```python
from build123d import *

# Parameters (mm, degrees)
SKETCH1_W           = 50.8
SKETCH1_H           = 25.4
SKETCH1_W_2         = 47.752
SKETCH1_H_2         = 22.352
EXTRUDE_THIN1_DEPTH = 304.8
SKETCH2_R           = 14.2875
CUT_EXTRUDE2_DEPTH  = 25.4


with BuildPart() as part:
    # Sketch1 → Extrude-Thin1 (new body)
    with BuildSketch(Plane.XY):
        with Locations((-25.4, -12.7)):
            Rectangle(SKETCH1_W, SKETCH1_H)
        with Locations((-25.4, -12.7)):
            Rectangle(SKETCH1_W_2, SKETCH1_H_2, mode=Mode.SUBTRACT)
    extrude(amount=EXTRUDE_THIN1_DEPTH)

    # Sketch2 → Cut-Extrude2 (cut)
    with BuildSketch(Plane(origin=(0, 0, 0), x_dir=(1, 0, 0), z_dir=(0, 1, 0))):
        with Locations(Location((-25.4, -25.4, 0), (0, 0, 270))):
            Circle(SKETCH2_R)
    extrude(amount=-CUT_EXTRUDE2_DEPTH, mode=Mode.SUBTRACT)


solid = part.part
```
Verification items for the finished model (mm, model axes). A direction names the side the tool comes from. Coordinates: 2 decimals unless noted, no trailing zeros. Write each loop counter-clockwise with the first axis right and the second up, starting at its lowest first coordinate (ties: lowest second). Pieces come first, ordered by that corner, then holes. Notation, with made-up numbers: (21.25, 73) - (40.25, 73) arc R22 cw to (40.25, 108) - close; hole circle Ø4 at (3, 54.5). An arc over 180 degrees is marked (long way). One line per question, with ' | ' between items. Start each with the question number.
1. Section check C-C (x = -17). Enter the section's corners in (y, z).
2. Section check B-B (z = 25.4). Enter the section's corners in (x, y).
3. Draft check along Z on faces 3 (the flat face through (-26, -25, 0)), 4 (the cylindrical face through (-15.744, -0.751, 14.87)), 5 (the flat face through (0, -13, 150)). Enter one of: released by +Z, released by -Z, zero draft, split by the parting line, or undercut.
4. Section check D-D (z = 219). Enter the section's corners in (x, y).
5. Access from +Z, -Z, +X, -X, +Y, -Y to the whole of each face (thin tool, end or side, straight path). Record for faces 1 (the cylindrical face through (-15.744, -24.627, 14.87)), 2 (the flat face through (-26, -23.876, 150)).
6. Section check A-A (y = -20). Enter the section's corners in (x, z), plus the area to 3 significant figures.
7. Material ranges on line 1 along X through (y, z) = (-7.25, 81.5); line 2 along Y through (x, z) = (-11.5, 33); line 3 along X through (y, z) = (-24.95, 25.4), recorded low to high.
Computed values:
1) outline: (-25.4, 0) - (-23.88, 0) - (-23.88, 13.84) - (-25.4, 13.84) - close; (-25.4, 36.96) - (-23.88, 36.96) - (-23.88, 304.8) - (-25.4, 304.8) - close; (-1.52, 0) - (0, 0) - (0, 13.84) - (-1.52, 13.84) - close; (-1.52, 36.96) - (0, 36.96) - (0, 304.8) - (-1.52, 304.8) - close
2) outline: (-50.8, -25.4) - (-39.69, -25.4) - (-39.69, -23.88) - (-49.28, -23.88) - (-49.28, -1.52) - (-39.69, -1.52) - (-39.69, 0) - (-50.8, 0) - close; (-11.11, -25.4) - (0, -25.4) - (0, 0) - (-11.11, 0) - (-11.11, -1.52) - (-1.52, -1.52) - (-1.52, -23.88) - (-11.11, -23.88) - close
3) face 3: released by -Z | face 4: undercut | face 5: zero draft
4) outline: (-50.8, -25.4) - (0, -25.4) - (0, 0) - (-50.8, 0) - close; hole (-49.28, -23.88) - (-1.52, -23.88) - (-1.52, -1.52) - (-49.28, -1.52) - close
5) face 1: +Y, -Y | face 2: +Z, -Z
6) outline: (-50.8, 0) - (-49.28, 0) - (-49.28, 304.8) - (-50.8, 304.8) - close; (-1.52, 0) - (0, 0) - (0, 304.8) - (-1.52, 304.8) - close | area: 929 mm²
7) line 1: -50.8 to -49.28, -1.52 to 0 | line 2: -25.4 to -23.88, -1.52 to 0 | line 3: -50.8 to -39.69, -11.11 to 0
